Design review of the part shown in the three views and the two pictorial views. Dimensions are in mm from the part's minimum x, y and z. Give positions to 0.01 mm unless a question says otherwise; leave off trailing zeros. Loops run counter-clockwise (first coordinate to the right, second up) from the corner with the lowest first, then second, coordinate; pieces in that order, holes last. Notation, with made-up numbers: (55.25, 21.25) - (77.25, 21.25) arc R27 cw to (77.25, 44.25) - close; hole circle Ø6 at (-5.5, 43). An arc over 180 degrees is marked (long way). Answer as a JSON object with one key per item and string values.
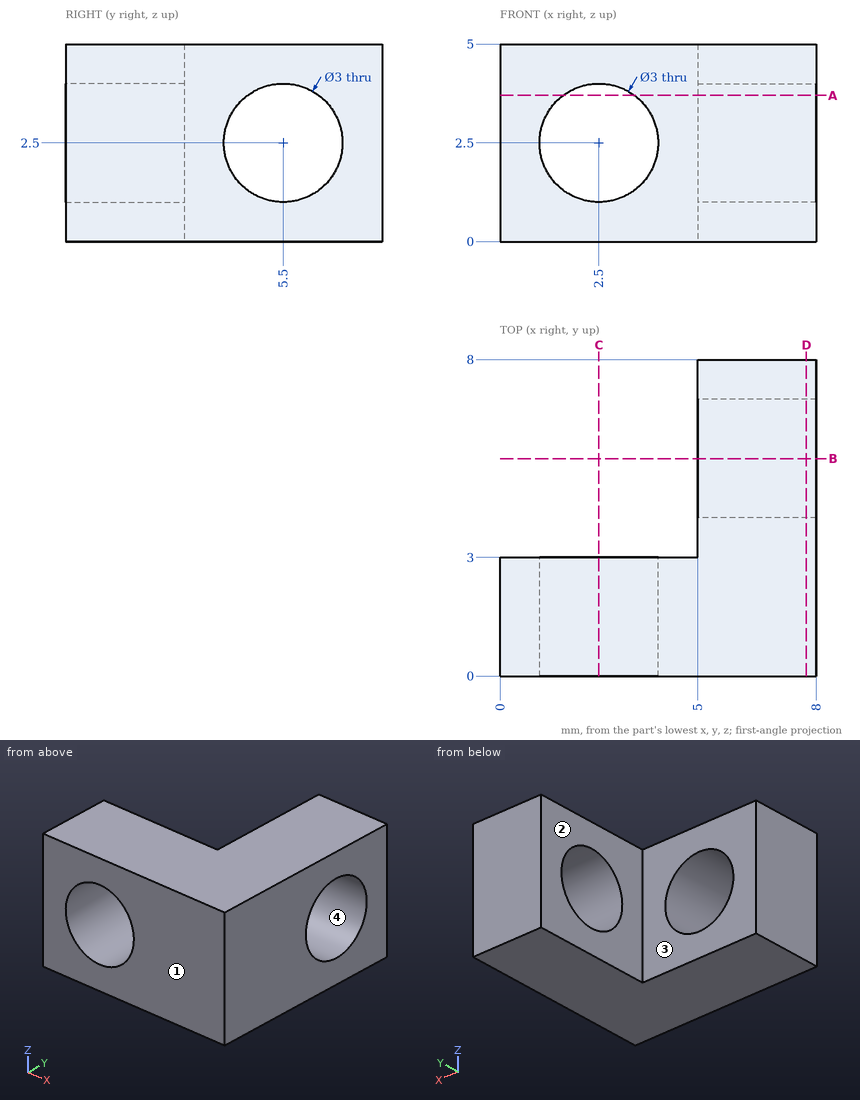
Q1. To check wall thickness, follow probe 1 along Y at (x, z) = (6.2, 2.5); probe 2 along Y at (x, z) = (1, 2.1); probe 3 along X at (y, z) = (0.7, 2.5). State the ranges of each line that lie inside material, in increasing order. Write a range as [from, to].
Results:
{"probe 1": "y = [0, 4], [7, 8]", "probe 2": "y = [0, 3]", "probe 3": "x = [0, 1], [4, 8]"}
Q2. Consider section A-A, the plane z = 3.7. State the section outline as (x, y) points.
Results:
{"outline": "(0, 0) - (1.6, 0) - (1.6, 3) - (0, 3) - close; (3.4, 0) - (8, 0) - (8, 4.6) - (5, 4.6) - (5, 3) - (3.4, 3) - close; (5, 6.4) - (8, 6.4) - (8, 8) - (5, 8) - close"}
Q3. The part is to be moulded in two halves that separate along Y. For the marked faces 1, 2, 3 and 4, say which applies: +Y half, -Y half, draft (parallel to the pull), parting line (faces both ways), or undercut.
Results:
{"face 1": "-Y half", "face 2": "draft", "face 3": "+Y half", "face 4": "undercut"}
Q4. Consider section C-C, the plane x = 2.5. State the section outline as (y, z) points.
Results:
{"outline": "(0, 0) - (3, 0) - (3, 1) - (0, 1) - close; (0, 4) - (3, 4) - (3, 5) - (0, 5) - close"}
Q5. Clearance check with a flat-ended pin moving along its axis: pin 1 Ø1.8 at (x, z) = (2.5, 2.5) entering from -Y. State where the tip first meets the part, or that it passes through.
Results:
{"pin 1": "passes through"}
Q6. Consider section D-D, the plane x = 7.75. State the section outline as (y, z) points, plus the area to 3 significant figures.
Results:
{"outline": "(0, 0) - (8, 0) - (8, 5) - (0, 5) - close; hole circle Ø3 at (5.5, 2.5)", "area": "32.9 mm^2"}
Q7. Consider section B-B, the plane y = 5.5. State the section outline as (x, z) points.
Results:
{"outline": "(5, 0) - (8, 0) - (8, 1) - (5, 1) - close; (5, 4) - (8, 4) - (8, 5) - (5, 5) - close"}
